```python
from build123d import *

# Parameters (mm, degrees)
SKETCH_1_R                   = 2
SKETCH_1_W                   = 70
SKETCH_1_H                   = 15
EXTRUDE_2_DEPTH              = 8
HOLE_WIZARD_M3_1_D           = 2.5
HOLE_WIZARD_M3_1_DEPTH       = 6.748924226
HOLE_WIZARD_M3_1_CSINK_D     = 3.05
HOLE_WIZARD_M3_1_CSINK_ANGLE = 45
HOLE_WIZARD_M3_1_TIP         = 0.751075774
HOLE_WIZARD_M3_2_D           = 2.5
HOLE_WIZARD_M3_2_DEPTH       = 6.748924226
HOLE_WIZARD_M3_2_CSINK_D     = 3.05
HOLE_WIZARD_M3_2_CSINK_ANGLE = 45
HOLE_WIZARD_M3_2_TIP         = 0.751075774
HOLE_WIZARD_M3_3_D           = 2.5
HOLE_WIZARD_M3_3_DEPTH       = 6.748924226
HOLE_WIZARD_M3_3_CSINK_D     = 3.05
HOLE_WIZARD_M3_3_CSINK_ANGLE = 45
HOLE_WIZARD_M3_3_TIP         = 0.751075774


with BuildPart() as part:
    # 草圖1 → 填料-伸長2 (new body)
    with BuildSketch(Plane.XY):
        Polygon((0, 0), (-50, 0), (-50, 35), (50, 35), (50, 0), align=None)
        with Locations((-21.5, 27.37)):
            Circle(SKETCH_1_R, mode=Mode.SUBTRACT)
        with Locations((21.5, 27.37)):
            Circle(SKETCH_1_R, mode=Mode.SUBTRACT)
        with Locations((0, 13.685)):
            Rectangle(SKETCH_1_W, SKETCH_1_H, mode=Mode.SUBTRACT)
    extrude(amount=EXTRUDE_2_DEPTH)

    # M3 螺紋孔1
    with Locations(Plane(origin=(50, 10, 4), x_dir=(0, 0, 1), z_dir=(1, 0, 0))):
        with Locations((0, 0), (0, -20), (0, -10)):
            CounterSinkHole(HOLE_WIZARD_M3_1_D / 2, HOLE_WIZARD_M3_1_CSINK_D / 2, depth=HOLE_WIZARD_M3_1_DEPTH, counter_sink_angle=HOLE_WIZARD_M3_1_CSINK_ANGLE)
            with Locations((0, 0, -(HOLE_WIZARD_M3_1_DEPTH + HOLE_WIZARD_M3_1_TIP / 2))):  # 118° drill point
                Cone(0, HOLE_WIZARD_M3_1_D / 2, HOLE_WIZARD_M3_1_TIP, mode=Mode.SUBTRACT)

    # M3 螺紋孔2
    with Locations(Plane(origin=(-50, 30, 4), x_dir=(0, 0, -1), z_dir=(-1, 0, 0))):
        with Locations((0, 0), (0, 10), (0, 20)):
            CounterSinkHole(HOLE_WIZARD_M3_2_D / 2, HOLE_WIZARD_M3_2_CSINK_D / 2, depth=HOLE_WIZARD_M3_2_DEPTH, counter_sink_angle=HOLE_WIZARD_M3_2_CSINK_ANGLE)
            with Locations((0, 0, -(HOLE_WIZARD_M3_2_DEPTH + HOLE_WIZARD_M3_2_TIP / 2))):  # 118° drill point
                Cone(0, HOLE_WIZARD_M3_2_D / 2, HOLE_WIZARD_M3_2_TIP, mode=Mode.SUBTRACT)

    # M3 螺紋孔3
    with Locations(Plane(origin=(40, 0, 4), x_dir=(-1, 0, 0), z_dir=(0, -1, 0))):
        with Locations((0, 0), (40, 0), (80, 0)):
            CounterSinkHole(HOLE_WIZARD_M3_3_D / 2, HOLE_WIZARD_M3_3_CSINK_D / 2, depth=HOLE_WIZARD_M3_3_DEPTH, counter_sink_angle=HOLE_WIZARD_M3_3_CSINK_ANGLE)
            with Locations((0, 0, -(HOLE_WIZARD_M3_3_DEPTH + HOLE_WIZARD_M3_3_TIP / 2))):  # 118° drill point
                Cone(0, HOLE_WIZARD_M3_3_D / 2, HOLE_WIZARD_M3_3_TIP, mode=Mode.SUBTRACT)


solid = part.part
```
Can you work these out from the model? Positions are in its coordinate system, mm. A direction names the side the tool comes from. Coordinates: 2 decimals unless noted, no trailing zeros. Loops run counter-clockwise (first coordinate to the right, second up) from the corner with the lowest first, then second, coordinate; pieces in that order, holes last. Notation, with made-up numbers: (68, 40.5) -> (94, 40.5) arc R25 cw to (94, 78.5) -> close; hole circle Ø7 at (-14.75, -4.75). An arc over 180 degrees is marked (long way). Put each result on its own line as item: value. Start each with the question number.
Q1. I want a section at D-D (y = 5). Write out the boundary of the cut face in (x, z), plus the area to 3 significant figures.
Q2. Thinking about a two-plate mould opening in Z: for faces 5 (the face through (-42.63, 9.99, 4.22)), 6 (the face through (1, 22, 0)), 7 (the face through (21.24, 29.353, 3.944)), which applies, pulls with the +Z half, pulls with the -Z half, needs draft (parallel to the pull), parting line crosses it, or undercut?
Q3. I want a section at C-C (x = -15). Write out the boundary of the cut face in (y, z) (3 decimals).
Q4. I want a section at B-B (y = 14). Write out the boundary of the cut face in (x, z).
Q5. For faces 1 (the face through (39.01, 3.75, 4.76)), 2 (the face through (-46.251, 8.946, 4.672)), 3 (the face through (-21.76, 29.353, 3.944)), 4 (the face through (46.25, 8.76, 4.16)), which set-ups out of +Z, -Z, +X, -X, +Y, -Y let a thin tool reach every point of the face, with its end or its side?
Q6. I want a section at A-A (x = 21.5). Write out the boundary of the cut face in (y, z) (3 decimals).
Q7. I'm going to push flat-ended pins straight in: P1, Ø2.5, axis at x = -21.5, y = 27.37, coming from the +Z side; P2, Ø2, axis at y = 20, z = 4, coming from the -X side; P3, Ø2, axis at y = 20, z = 4, coming from the +X side; P4, Ø1.5, axis at y = 30, z = 4, coming from the -X side. Where does each tip first touch, or does it pass through?
Q8. If I drill on line 1 (Y direction, x = 48, z = 4); line 2 (X direction, y = 4.75, z = 4); line 3 (Y direction, x = 4.5, z = 1.5) (3 decimals), over which ranges is the centre line in solid material (lowest first)? Write a range as [from, to].
Taken from the geometry:
1. outline: (-50, 0) -> (50, 0) -> (50, 8) -> (-50, 8) -> close; hole circle Ø2.5 at (-40, 4); hole circle Ø2.5 at (0, 4); hole circle Ø2.5 at (40, 4)
1. area: 785 mm2
2. face 5: undercut
2. face 6: pulls with the -Z half
2. face 7: needs draft
3. outline: (0, 0) -> (6.185, 0) -> (6.185, 8) -> (0, 8) -> close; (21.185, 0) -> (35, 0) -> (35, 8) -> (21.185, 8) -> close
4. outline: (-50, 0) -> (-35, 0) -> (-35, 8) -> (-50, 8) -> close; (35, 0) -> (50, 0) -> (50, 8) -> (35, 8) -> close
5. face 1: -Y
5. face 2: -X
5. face 3: +Z, -Z
5. face 4: +X
6. outline: (0, 0) -> (6.185, 0) -> (6.185, 8) -> (0, 8) -> close; (21.185, 0) -> (25.37, 0) -> (25.37, 8) -> (21.185, 8) -> close; (29.37, 0) -> (35, 0) -> (35, 8) -> (29.37, 8) -> close
7. P1: passes through
7. P2: stops at x = -43.1
7. P3: stops at x = 43.1
7. P4: stops at x = -42.95
8. line 1: y = [0, 8.75], [11.25, 18.75], [21.25, 28.75], [31.25, 35]
8. line 2: x = [-50, -41.25], [-38.75, -1.25], [1.25, 38.75], [41.25, 50]
8. line 3: y = [0, 6.185], [21.185, 35]
